Work out the finished part from the listing and answer in its coordinate system (mm). Coordinates: 2 decimals unless noted, no trailing zeros. Order: outer loops, then holes, each group sorted by start corner. A loop starts at its lowest first (then second) coordinate and runs counter-clockwise, first axis right, second up.
Autodesk Inventor part; units mm, degrees
ref_plane "YZ Plane" through (0, 0, 0) normal (1, 0, 0) x (0, 1, 0)
ref_plane "XZ Plane" through (0, 0, 0) normal (0, 1, 0) x (-1, 0, 0)
ref_plane "XY Plane" through (0, 0, 0) normal (0, 0, 1) x (1, 0, 0)
sketch "Sketch1" plane through (0, 0, 0) normal (0, 0, 1) x (1, 0, 0)
  line L0 (-150, -75) -> (150, -75)
  line L1 (150, -75) -> (150, 75)
  line L2 (150, 75) -> (-150, 75)
  line L3 (-150, 75) -> (-150, -75)
  line L4 (-150, -75) -> (150, 75) construction
  line L5 (150, -75) -> (-150, 75) construction
  point P0 (0, 0)
  dimension "d0" = 300
  dimension "d1" = 150
extrude "Extrusion1" add sketch "Sketch1" along normal blind 25.4
sketch "Sketch2" plane through (0, 0, 25.4) normal (0, 0, 1) x (1, 0, 0)
  line L0 (-120, 0) -> (120, 0)
  line L1 (-150, 75) -> (-150, -75)
  point P0 (0, 0)
  point P1 (0, 0)
  dimension "d4" = 30
hole "Hole1" at (-120, 0, 25.4) at (120, 0, 25.4) direction (0, 0, -1) diameter 10 end through all
sketch "Sketch3" plane through (0, 0, 25.4) normal (0, 0, 1) x (1, 0, 0)
  line L0 (-93, 0) -> (93, 0)
  point P0 (0, 0)
  point P1 (0, 0)
  dimension "d38" = 186
hole "Hole2" at (-93, 0, 25.4) at (93, 0, 25.4) direction (0, 0, -1) diameter 8 end through all
sketch "Sketch5" plane through (0, 0, 25.4) normal (0, 0, 1) x (1, 0, 0)
  line L0 (0, 0) -> (150, 0)
  line L1 (150, -75) -> (150, 75)
  circle A0 centre (47.5, 0) radius 2
  circle A1 centre (62.5, 0) radius 2
  dimension "d26" = 4
  dimension "d27" = 47.5
  dimension "d37" = 15
extrude "Extrusion2" cut sketch "Sketch5" against normal through all
pattern_linear "Rectangular Pattern1" count 2 spacing 15 along (0, -1, 0) count 2 spacing -15 along (0, -1, 0) of "Extrusion2"
properties part number "base de madera pequeña"
1. The mould has two halves that part along Y. Classify faces 1 (the flat face through (-2, 1, 25.4)), 2 (the flat face through (2, 75, 13)), 3 (the cylindrical face through (116, -3, 13)): released by +Y, released by -Y, zero draft, split by the parting line, or undercut.
2. The part is cut by section A-A (x = -120). Determine the outline of the cut face in (y, z).
3. A flat-ended cylindrical pin translates along its axis: pin 1 (9 mm diameter, centred on x = 120, y = 0, fed in from +Z). Find the tip coordinate at first contact, or state that the pin passes through.
4. Consider probe 1 along Y at (x, z) = (47.5, 8); probe 2 along Y at (x, z) = (-93, 14.25); probe 3 along Y at (x, z) = (-120, 11.75). Determine where each line is inside the solid, lowest interval first.
Worked out:
1. face 1: zero draft
1. face 2: released by +Y
1. face 3: undercut
2. outline: (-75, 0) - (-5, 0) - (-5, 25.4) - (-75, 25.4) - close; (5, 0) - (75, 0) - (75, 25.4) - (5, 25.4) - close
3. pin 1: passes through
4. probe 1: y = -75 to -17, -13 to -2, 2 to 13, 17 to 75
4. probe 2: y = -75 to -4, 4 to 75
4. probe 3: y = -75 to -5, 5 to 75
